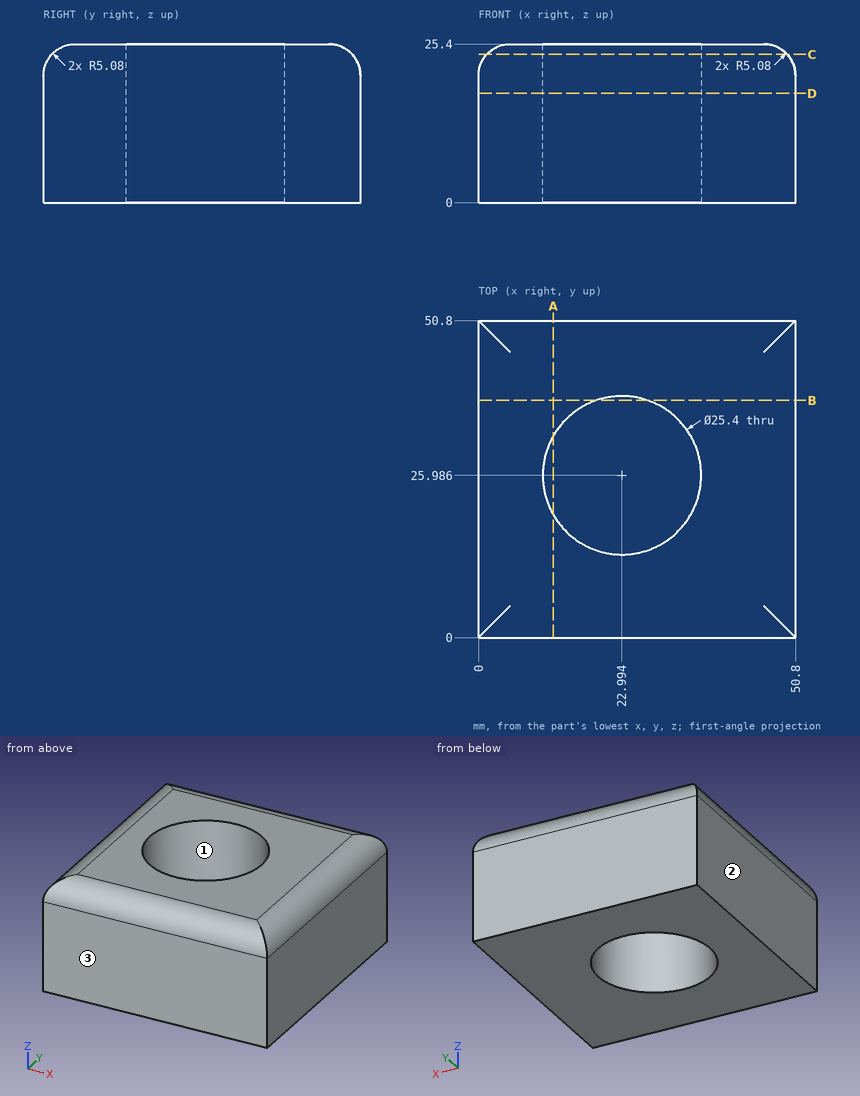
Can you work these out from the drawing? Everything is in mm from the part's minimum corner. Coordinates: 2 decimals unless noted, no trailing zeros. Loops run counter-clockwise (first coordinate to the right, second up) from the corner with the lowest first, then second, coordinate; pieces in that order, holes last.
1) Will this pin go through, and if not, where does the flat tip stop? pin 1 Ø2 at (y, z) = (31, 6) entering from -X.
Reported:
pin 1: stops at x = 0
2) Imagine slicing it at C-C (z = 23.75). List the corners of the cut face in (x, y) for me (1 decimal), and give its area (3 significant figures).
Reported:
outline: (1.3, 1.3) - (49.5, 1.3) - (49.5, 49.5) - (1.3, 49.5) - close; hole circle Ø25.4 at (23, 26)
area: 1,810 mm2
3) Thinking about a two-plate mould opening in Y: for the marked faces 1, 2 and 3, which applies, released by +Y, released by -Y, zero draft, split by the parting line, or undercut?
Reported:
face 1: undercut
face 2: zero draft
face 3: released by -Y
4) Please list where these lines run through material, in increasing order: line 1 along Y through (x, z) = (31, 7.5) (1 decimal); line 2 along Y through (x, z) = (16, 17) (1 decimal); line 3 along X through (y, z) = (31.5, 14.5) (1 decimal).
Reported:
line 1: y = 0 to 16.1, 35.8 to 50.8
line 2: y = 0 to 15.4, 36.6 to 50.8
line 3: x = 0 to 11.6, 34.4 to 50.8
5) Imagine slicing it at B-B (y = 38). List the corners of the cut face in (x, z) for me.
Reported:
outline: (0, 0) - (18.88, 0) - (18.88, 25.4) - (5.08, 25.4) arc R5.08 ccw to (0, 20.32) - close; (27.11, 0) - (50.8, 0) - (50.8, 20.32) arc R5.08 ccw to (45.72, 25.4) - (27.11, 25.4) - close
6) Imagine slicing it at D-D (z = 17.5). List the corners of the cut face in (x, y) for me (1 decimal).
Reported:
outline: (0, 0) - (50.8, 0) - (50.8, 50.8) - (0, 50.8) - close; hole circle Ø25.4 at (23, 26)
7) Imagine slicing it at A-A (x = 12). List the corners of the cut face in (y, z) for me, and give its area (3 significant figures).
Reported:
outline: (0, 0) - (19.63, 0) - (19.63, 25.4) - (5.08, 25.4) arc R5.08 ccw to (0, 20.32) - close; (32.34, 0) - (50.8, 0) - (50.8, 20.32) arc R5.08 ccw to (45.72, 25.4) - (32.34, 25.4) - close
area: 956 mm2
